Autodesk Inventor part; units mm, degrees
ref_plane "WorkPlane1" through (0, 0, 0) normal (0, 0, 1) x (1, 0, 0)
ref_plane "WorkPlane3" through (0, 0, -7.54) normal (0, 0, 1) x (1, 0, 0)
ref_plane "Work Plane3" through (0, -24.68, 0) normal (0, 1, 0) x (-1, 0, 0)
ref_plane "WorkPlane1" through (0, 0, 0) normal (0, 0, 1) x (1, 0, 0)
ref_plane "WorkPlane3" through (0, 0, -7.54) normal (0, 0, 1) x (1, 0, 0)
ref_plane "Work Plane3" through (0, -24.68, 0) normal (0, 1, 0) x (-1, 0, 0)
ref_plane "WorkPlane10" through (0, 24.68, 0) normal (0, 1, 0) x (-1, 0, 0)
sketch "Sketch1" plane through (0, 0, 0) normal (0, 0, 1) x (1, 0, 0)
  point P0 (0, 0)
sketch "Sketch2" plane through (0, 0, 0) normal (0, 0, 1) x (1, 0, 0)
  circle A0 centre (0, 0) radius 24.68
  dimension "d3" = 49.36
extrude "Extrusion1" add sketch "Sketch2" against normal blind 7.54
sketch "Sketch3" plane through (0, 0, -7.54) normal (0, 0, 1) x (1, 0, 0)
  point P0 (0, 0)
sketch "Sketch4" plane through (0, 0, 0) normal (0, 0, 1) x (1, 0, 0)
  circle A0 centre (0, 0) radius 24.68
hole "Hole1" at (0, 0, 0) direction (0, 0, -1) diameter 31.25 end through all
sketch "Sketch5" plane through (0, 24.68, 0) normal (0, 1, 0) x (-1, 0, 0)
  line L0 (-0.387, 0) -> (-2.272, 0)
  line L1 (0.9425, -7.54) -> (-0.387, 0)
  line L2 (-0.9425, -7.54) -> (0.9425, -7.54)
  line L3 (-2.272, 0) -> (-0.9425, -7.54)
  line L4 (-15.625, 0) -> (15.625, 0) construction
  line L5 (24.68, -7.54) -> (-24.68, -7.54) construction
  line L6 (0, -9.048) -> (0, 1.508)
  dimension "d15" = 80
  dimension "d18" = 0.9425
  dimension "d19" = 0.9425
extrude "Extrusion2" cut sketch "Sketch5" against normal blind 24.68
ref_plane "MSC_PT1" through (0, 0, 0) normal (0, 0, 1) x (1, 0, 0)
ref_plane "MSC_PT2" through (0, 0, -7.54) normal (0, 0, -1) x (-1, 0, 0)
equation "\"d7\" = Diam1"
equation "\"d4\" = ParH"
equation "\"d18\" = 0.125 * ParH"
equation "\"d19\" = 0.125 * ParH"
equation "\"d16\" = 0.5 * Diam2"
equation "\"d3\" = Diam2"
equation "\"Diam2\" = 49.36"
equation "\"ParH\" = 7.54"
equation "\"Diam1\" = 31.25"
equation "\"d20\" = 0.5 * Diam2"
properties part number "ASME B18.21.2M - 30" material "Steel, Mild"
Geometry: final body of the model. Coordinates: model frame, mm. A direction names the side the tool comes from. Coordinates: 2 decimals unless noted, no trailing zeros. Loops run counter-clockwise (first coordinate to the right, second up) from the corner with the lowest first, then second, coordinate; pieces in that order, holes last. Notation, with made-up numbers: M -12.75,9 L 37.25,9 A21 ccw 37.25,32 Z; hole C 73,40.25 d5. An arc over 180 degrees is marked long. One line per item, written item: value. Start each with the question number.
1) Cut plane B-B (x = -4). Return loops of the section in (y, z).
2) Draft query along X for faces 1 (the flat face through (-0.287, 20.202, -3.823)), 2 (the flat face through (0, -16, 0)). Return one class per face: released by +X, released by -X, zero draft, split by the parting line, or undercut.
3) Cut plane A-A (y = 8.5). Return loops of the section in (x, z).
4) Pin query (flat end, axial travel): P1, Ø12, axis at x = -1, y = -7, coming from the -Z side; P2, Ø5, axis at x = 4, y = -13.5, coming from the +Z side; P3, Ø1.5, axis at y = -1, z = -3.5, coming from the -X side; P4, Ø2, axis at x = -19, z = -3, coming from the -Y side (3 decimals). Return the tip coordinate at first contact, or that it passes through.
5) Cut plane C-C (z = -5.75). Return loops of the section in (x, y) (3 decimals), then the cut area to 3 significant figures.
6) Reachability of faces 3 (the flat face through (1.617, 20.125, -3.717)), 4 (the flat face through (0, -16, -7.54)) from +Z, -Z, +X, -X, +Y, -Y: full face, straight path, thin tool, end or side. Return the list, or none.
7) Cut plane D-D (x = -21.5). Return loops of the section in (y, z), then the cut area to 3 significant figures.
8) Material intervals for L1, parallel to X at y = 12, z = -6.75; L2, parallel to X at y = 20, z = -5.5; L3, parallel to Y at x = -13.5, z = -5.5, sorted ascending. Write a range as from..to.
Evaluation:
1. outline: M -24.35,-7.54 L -15.1,-7.54 L -15.1,0 L -24.35,0 Z; M 15.1,-7.54 L 24.35,-7.54 L 24.35,0 L 15.1,0 Z
2. face 1: undercut
2. face 2: zero draft
3. outline: M -23.17,-7.54 L -13.11,-7.54 L -13.11,0 L -23.17,0 Z; M 13.11,-7.54 L 23.17,-7.54 L 23.17,0 L 13.11,0 Z
4. P1: through
4. P2: z = 0
4. P3: x = -24.68
4. P4: y = -16.885
5. outline: M -0.627,15.612 L -0.627,24.672 A24.68 ccw long 1.258,24.648 L 1.258,15.574 A15.625 cw long Z
5. area: 1,130 mm^2
6. face 3: +Z, +Y
6. face 4: -Z, +X, -X, +Y, -Y
7. outline: M -12.12,-7.54 L 12.12,-7.54 L 12.12,0 L -12.12,0 Z
7. area: 183 mm^2
8. L1: -21.57..-10.01, 10.01..21.57
8. L2: -14.46..-0.58, 1.3..14.46
8. L3: -20.66..-7.87, 7.87..20.66
